Can you work these out from the model? Positions are in its coordinate system, mm. Face numbers are marked on the shaded views. A direction names the side the tool comes from. Give positions to 0.01 mm unless a question says otherwise; leave off trailing zeros. Loops run counter-clockwise (first coordinate to the right, second up) from the corner with the lowest first, then second, coordinate; pieces in that order, holes last. Notation, with made-up numbers: M 29,-25 L 50,-25 A14 cw 50,-21 Z; hole C -18.75,74 d11. An arc over 180 degrees is marked long. Use CSV: the item, a comma, the result in double quotes.
from build123d import *

# Parameters (mm, degrees)
BOSS_EXTRU_1_DEPTH        = 13
COQUE1_T                  = -5
COQUE1_THICKNESS_2_FACE_W = 65
COQUE1_THICKNESS_2_FACE_H = 65
COQUE1_THICKNESS_2_DEPTH  = 2
ENL_V_MAT_EXTRU_1_REACH   = 88.587
ESQUISSE2_R               = 2.5
ENL_V_MAT_EXTRU_2_REACH   = 95.396
ESQUISSE3_R               = 2.5
ESQUISSE4_W               = 18
ESQUISSE4_H               = 18
ESQUISSE4_W_2             = 15
ESQUISSE4_H_2             = 15
BOSS_EXTRU_2_DEPTH        = 10
ESQUISSE5_R               = 11.5
ESQUISSE5_R_2             = 14.5
ENL_V_MAT_EXTRU_3_DEPTH   = 13


with BuildPart() as part:
    # Esquisse1 → Boss.-Extru.1 (new body)
    with BuildSketch(Plane.XY):
        Polygon((44.118436308, 33.728448276), (54.118436308, 33.728448276), (54.118436308, 23.728448276), (54.118436308, -41.271551724), (-20.881563692, -41.271551724), (-20.881563692, 33.728448276), align=None)
    extrude(amount=BOSS_EXTRU_1_DEPTH)

    # Coque1
    coque1_openings = [part.faces().sort_by_distance(p)[0] for p in [
        (16.618436308, -3.771551724, 13),
    ]]
    offset(amount=COQUE1_T, openings=coque1_openings, kind=Kind.INTERSECTION)

    # Coque1 thickness 2 face (on inner face of the shell) → Coque1 thickness 2 (cut)
    with BuildSketch(Plane(origin=(16.618436308, -3.771551724, 5), x_dir=(-1, 0, 0), z_dir=(0, 0, -1))):
        Rectangle(COQUE1_THICKNESS_2_FACE_W, COQUE1_THICKNESS_2_FACE_H)
    extrude(amount=COQUE1_THICKNESS_2_DEPTH, mode=Mode.SUBTRACT)

    # Enlèv. mat.-Extru.1: up to this face of the body (flat: up to its plane)
    enl_v_mat_extru_1_end = Plane(part.part.faces().sort_by_distance((54.118436308, -3.771551724, 6.5))[0])
    # Esquisse2 → Enlèv. mat.-Extru.1 (cut, up to the picked face)
    with BuildSketch(Plane.ZY.offset(20.881563692), mode=Mode.PRIVATE) as enl_v_mat_extru_1_sk1:
        with Locations(Location((8, -16.271551724, 0), (0, 0, 270))):
            Circle(ESQUISSE2_R)
    enl_v_mat_extru_1_tool1 = split(extrude(enl_v_mat_extru_1_sk1.sketch, amount=-ENL_V_MAT_EXTRU_1_REACH, mode=Mode.PRIVATE), bisect_by=enl_v_mat_extru_1_end, keep=Keep.BOTH, mode=Mode.PRIVATE)
    # Esquisse2 → Enlèv. mat.-Extru.1 (cut, up to the picked face)
    with BuildSketch(Plane.ZY.offset(20.881563692), mode=Mode.PRIVATE) as enl_v_mat_extru_1_sk2:
        with Locations(Location((8, 8.728448276, 0), (0, 0, 270))):
            Circle(ESQUISSE2_R)
    enl_v_mat_extru_1_tool2 = split(extrude(enl_v_mat_extru_1_sk2.sketch, amount=-ENL_V_MAT_EXTRU_1_REACH, mode=Mode.PRIVATE), bisect_by=enl_v_mat_extru_1_end, keep=Keep.BOTH, mode=Mode.PRIVATE)
    add(enl_v_mat_extru_1_tool1.solids().sort_by(Axis((-20.881564, -16.271552, 8), (1, 0, 0)))[0], mode=Mode.SUBTRACT)
    add(enl_v_mat_extru_1_tool2.solids().sort_by(Axis((-20.881564, 8.728448, 8), (1, 0, 0)))[0], mode=Mode.SUBTRACT)

    # Enlèv. mat.-Extru.2: up to this face of the body (flat: up to its plane)
    enl_v_mat_extru_2_end = Plane(part.part.faces().sort_by_distance((16.618436308, 33.728448276, 6.5))[0])
    # Esquisse3 → Enlèv. mat.-Extru.2 (cut, up to the picked face)
    with BuildSketch(Plane.XZ.offset(41.271551724), mode=Mode.PRIVATE) as enl_v_mat_extru_2_sk1:
        with Locations(Location((4.118436308, 8, 0), (0, 0, 270))):
            Circle(ESQUISSE3_R)
    enl_v_mat_extru_2_tool1 = split(extrude(enl_v_mat_extru_2_sk1.sketch, amount=-ENL_V_MAT_EXTRU_2_REACH, mode=Mode.PRIVATE), bisect_by=enl_v_mat_extru_2_end, keep=Keep.BOTH, mode=Mode.PRIVATE)
    # Esquisse3 → Enlèv. mat.-Extru.2 (cut, up to the picked face)
    with BuildSketch(Plane.XZ.offset(41.271551724), mode=Mode.PRIVATE) as enl_v_mat_extru_2_sk2:
        with Locations(Location((29.118436308, 8, 0), (0, 0, 270))):
            Circle(ESQUISSE3_R)
    enl_v_mat_extru_2_tool2 = split(extrude(enl_v_mat_extru_2_sk2.sketch, amount=-ENL_V_MAT_EXTRU_2_REACH, mode=Mode.PRIVATE), bisect_by=enl_v_mat_extru_2_end, keep=Keep.BOTH, mode=Mode.PRIVATE)
    add(enl_v_mat_extru_2_tool1.solids().sort_by(Axis((4.118436, -41.271552, 8), (0, 1, 0)))[0], mode=Mode.SUBTRACT)
    add(enl_v_mat_extru_2_tool2.solids().sort_by(Axis((29.118436, -41.271552, 8), (0, 1, 0)))[0], mode=Mode.SUBTRACT)

    # Esquisse4 → Boss.-Extru.2 (add)
    with BuildSketch(Plane.XY.offset(3)):
        Polygon((-15.881563692, -26.271551724), (-5.881563692, -36.271551724), (-15.881563692, -36.271551724), align=None)
        with Locations((45.118436308, 24.728448276)):
            Rectangle(ESQUISSE4_W, ESQUISSE4_H)
        Polygon((49.118436308, -36.271551724), (49.118436308, -26.271551724), (39.118436308, -36.271551724), align=None)
        with Locations((-8.381563692, 21.228448276)):
            Rectangle(ESQUISSE4_W_2, ESQUISSE4_H_2)
    extrude(amount=BOSS_EXTRU_2_DEPTH)

    # Esquisse5 → Enlèv. mat.-Extru.3 (cut)
    with BuildSketch(Plane.XY.offset(13)):
        with Locations((-20.881563692, 33.728448276)):
            Circle(ESQUISSE5_R)
        with Locations((54.118436308, 33.728448276)):
            Circle(ESQUISSE5_R_2)
    extrude(amount=-ENL_V_MAT_EXTRU_3_DEPTH, mode=Mode.SUBTRACT)


solid = part.part
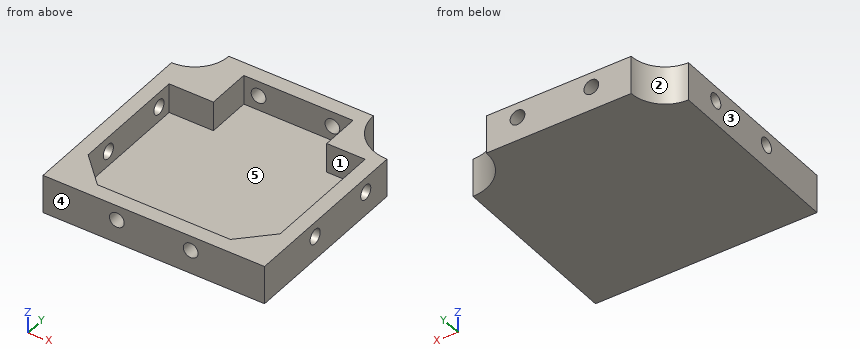
Q1. I want a section at C-C, the plane y = 4. Please give me the cut outline in (x, z), then the cut area to 3 significant figures.
Model answer:
outline,"M -20.88,0 L 54.12,0 L 54.12,13 L 49.12,13 L 49.12,3 L -15.88,3 L -15.88,13 L -20.88,13 Z"
area,"325 mm2"
Q2. I want a section at A-A, the plane x = 10.5. Please give me the cut outline in (y, z).
Model answer:
outline,"M -41.27,0 L 33.73,0 L 33.73,13 L 28.73,13 L 28.73,3 L -36.27,3 L -36.27,13 L -41.27,13 Z"
Q3. I'm going to push a flat-ended pin straight in: P1, Ø4, axis at y = -16.27, z = 8, coming from the +X side. Where does the tip first touch, or does it pass through?
Model answer:
P1,"through"
Q4. I want a section at B-B, the plane z = 4.5. Please give me the cut outline in (x, y).
Model answer:
outline,"M -20.88,-41.27 L 54.12,-41.27 L 54.12,19.23 A14.5 cw 39.62,33.73 L -9.38,33.73 A11.5 cw -20.88,22.23 Z; hole M -15.88,-26.27 L -5.88,-36.27 L 39.12,-36.27 L 49.12,-26.27 L 49.12,15.73 L 36.12,15.73 L 36.12,28.73 L -0.88,28.73 L -0.88,13.73 L -15.88,13.73 Z"
Q5. For the marked faces 1 and 2, which set-ups out of +Z, -Z, +X, -X, +Y, -Y let a thin tool reach every point of the face, with its end or its side?
Model answer:
face 1,"+Z"
face 2,"+Z, -Z, -X, +Y"
Q6. Please list where these lines run through material, in increasing order: L1, parallel to Y at x = 12.5, z = 8.25; L2, parallel to X at y = -23, z = 9; L3, parallel to Z at x = 51, y = -16. Write a range as from..to.
Model answer:
L1,"-41.27..-36.27, 28.73..33.73"
L2,"-20.88..-15.88, 49.12..54.12"
L3,"0..5.51, 10.49..13"
Q7. If we mould it in two halves opening along Y, with no side actions, what happens to the marked faces 3, 4 and 5? For each: released by +Y, released by -Y, zero draft, split by the parting line, or undercut.
Model answer:
face 3,"zero draft"
face 4,"released by -Y"
face 5,"undercut"
